Can you work these out from the drawing? Everything is in mm from the part's minimum corner. Round coordinates to 2 decimals unless told otherwise and drop trailing zeros. Order: outer loops, then holes, each group sorted by start corner. A loop starts at its lowest first (then second) coordinate and runs counter-clockwise, first axis right, second up. Notation, with made-up numbers: M 36.5,69 L 68.5,69 A18 cw 68.5,81 Z; hole C 11.25,4.25 d10. An arc over 180 degrees is marked long. Write each question's results on one line, items separated by ' | '. Start each with the question number.
1. I'm going to push flat-ended pins straight in: pin 1 (1.5 mm diameter, centred on x = 2, y = 31.5, fed in from +Z); pin 2 (3 mm diameter, centred on x = 3, y = 37.5, fed in from -Z); pin 3 (3 mm diameter, centred on x = 3.5, z = 47.5, fed in from -Y). Where does each tip first touch, or does it pass through?
2. Please list where these lines run through material, in increasing order: L1, parallel to Y at x = 1.25, z = 15.5 (3 decimals); L2, parallel to Y at x = 2, z = 73.
3. Suppose I cut it at B-B on z = 42. Write out the boundary of the cut face in (x, y) (3 decimals), and give its area (3 significant figures).
4. Suppose I cut it at D-D on y = 61. Write out the boundary of the cut face in (x, z).
5. Suppose I cut it at A-A on y = 69. Write out the boundary of the cut face in (x, z), and give its area (3 significant figures).
6. Suppose I cut it at C-C on x = 2.5. Write out the boundary of the cut face in (y, z) (3 decimals), and give its area (3 significant figures).
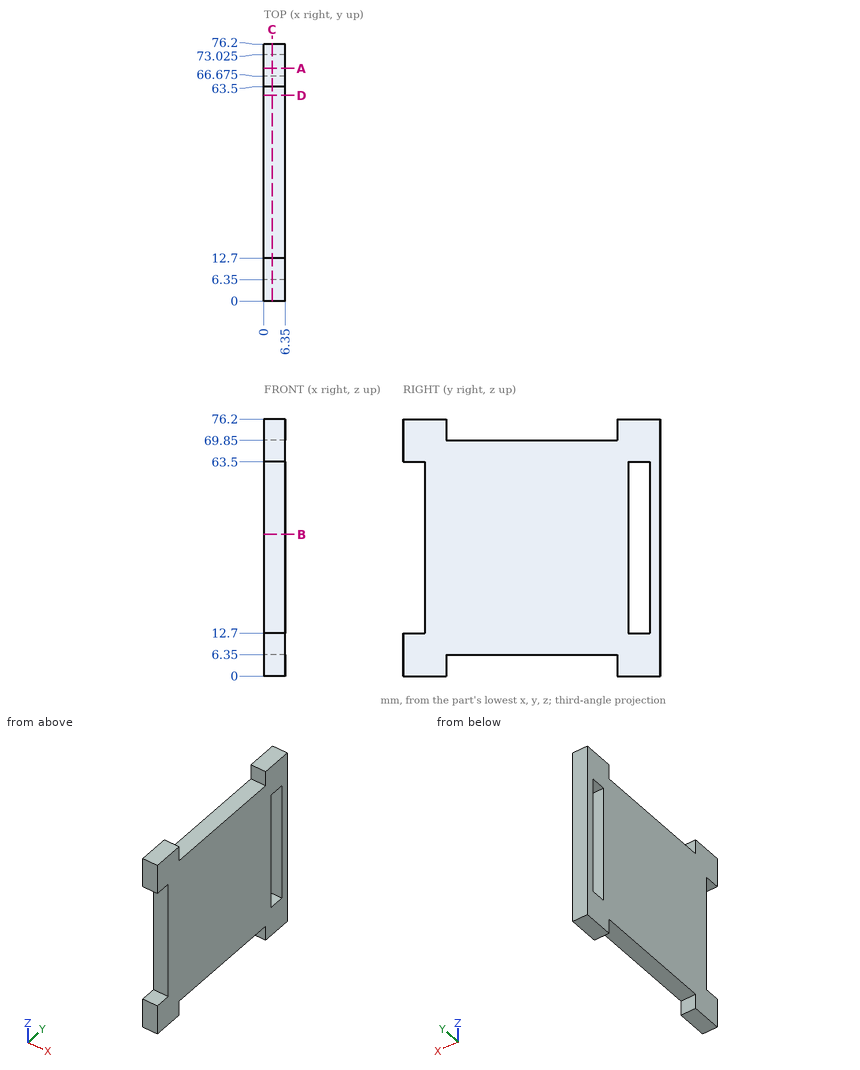
Filled sheet:
1) pin 1: stops at z = 69.85 | pin 2: stops at z = 6.35 | pin 3: stops at y = 6.35
2) L1: y = 6.35 to 66.675, 73.025 to 76.2 | L2: y = 0 to 12.7, 63.5 to 76.2
3) outline: M 0,6.35 L 6.35,6.35 L 6.35,66.675 L 0,66.675 Z; M 0,73.025 L 6.35,73.025 L 6.35,76.2 L 0,76.2 Z | area: 403 mm^2
4) outline: M 0,6.35 L 6.35,6.35 L 6.35,69.85 L 0,69.85 Z
5) outline: M 0,0 L 6.35,0 L 6.35,12.7 L 0,12.7 Z; M 0,63.5 L 6.35,63.5 L 6.35,76.2 L 0,76.2 Z | area: 161 mm^2
6) outline: M 0,0 L 12.7,0 L 12.7,6.35 L 63.5,6.35 L 63.5,0 L 76.2,0 L 76.2,76.2 L 63.5,76.2 L 63.5,69.85 L 12.7,69.85 L 12.7,76.2 L 0,76.2 L 0,63.5 L 6.35,63.5 L 6.35,12.7 L 0,12.7 Z; hole M 66.675,12.7 L 73.025,12.7 L 73.025,63.5 L 66.675,63.5 Z | area: 4,520 mm^2
